Could you check a few things on this model? Use its own coordinates, in mm. Face numbers are marked on the shaded views. A direction names the side the tool comes from. Round coordinates to 2 decimals unless told otherwise and drop trailing zeros. Write each loop counter-clockwise with the first axis right and the second up, starting at its lowest first coordinate (ties: lowest second). Pieces come first, ordered by that corner, then holes. Notation, with made-up numbers: (9, -33.5) -> (31, -33.5) arc R35 cw to (31, 4.5) -> close; hole circle Ø10 at (12.25, 33). An arc over 180 degrees is marked (long way). Answer in a Markdown table with one row per item.
from build123d import *

# Parameters (mm, degrees)
SKETCH1_R           = 3
BOSS_EXTRUDE1_DEPTH = 1
BOSS_EXTRUDE2_DEPTH = 4
SKETCH3_R           = 1.5
BOSS_EXTRUDE3_DEPTH = 8
CHAMFER1_SIZE       = 0.5
SKETCH4_R           = 1.5
CUT_EXTRUDE1_DEPTH  = 3


with BuildPart() as part:
    # Sketch1 → Boss-Extrude1 (new body)
    with BuildSketch(Plane(origin=(0, 0, 0), x_dir=(1, 0, 0), z_dir=(0, 1, 0))):
        with Locations(Location((0, 0, 0), (0, 0, 270))):
            Circle(SKETCH1_R)
    extrude(amount=BOSS_EXTRUDE1_DEPTH)

    # Sketch2 → Boss-Extrude2 (add)
    with BuildSketch(Plane(origin=(0, 1, 0), x_dir=(1, 0, 0), z_dir=(0, 1, 0))):
        Polygon((3.464101615, 0), (1.732050808, 3), (-1.732050808, 3), (-3.464101615, 0), (-1.732050808, -3), (1.732050808, -3), align=None)
    extrude(amount=BOSS_EXTRUDE2_DEPTH)

    # Sketch3 → Boss-Extrude3 (add)
    with BuildSketch(Plane(origin=(0, 5, 0), x_dir=(1, 0, 0), z_dir=(0, 1, 0))):
        with Locations(Location((0, 0, 0), (0, 0, 270))):
            Circle(SKETCH3_R)
    extrude(amount=BOSS_EXTRUDE3_DEPTH)

    # Chamfer1
    chamfer1_edges = [part.edges().sort_by_distance(p)[0] for p in [
        (0, 13, -1.5),
    ]]
    chamfer(chamfer1_edges, length=CHAMFER1_SIZE)

    # Sketch4 → Cut-Extrude1 (cut)
    with BuildSketch(Plane.XZ):
        with Locations(Location((0, 0, 0), (0, 0, 90))):
            Circle(SKETCH4_R)
    extrude(amount=-CUT_EXTRUDE1_DEPTH, mode=Mode.SUBTRACT)


solid = part.part
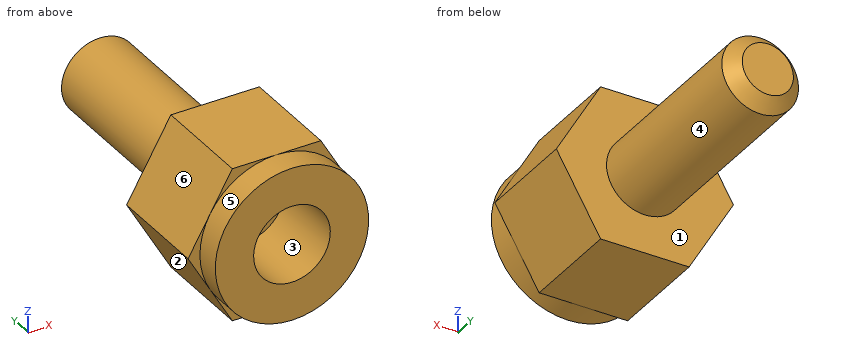
1) Imagine slicing it at D-D, the plane y = 8.5. Please give me the cut outline in (x, z), plus the area to 3 significant figures.
Findings:
| item | result |
|---|---|
| outline | circle Ø3 at (0, 0) |
| area | 7.07 mm^2 |
2) For pin 1 (1.5 mm diameter, centred on x = -1.5, z = -2.5, fed in from +Y), with a flat end and sliding along its axis, tell me the tip position at first contact or that it passes through.
Findings:
| item | result |
|---|---|
| pin 1 | stops at y = 5 |
3) Thinking about a two-plate mould opening in Z: for the marked faces 1, 2 and 3, which applies, +Z half, -Z half, draft (parallel to the pull), parting line (faces both ways), or undercut?
Findings:
| item | result |
|---|---|
| face 1 | draft |
| face 2 | -Z half |
| face 3 | undercut |
4) For the marked faces 4, 5 and 6, which set-ups out of +Z, -Z, +X, -X, +Y, -Y let a thin tool reach every point of the face, with its end or its side?
Findings:
| item | result |
|---|---|
| face 4 | +Y |
| face 5 | -Y |
| face 6 | +Z, -X, +Y, -Y |
5) Please list where these lines run through material, in increasing order: line 1 (X direction, y = 0.75, z = 0); line 2 (Y direction, x = 0, z = 0.5); line 3 (Y direction, x = -1, z = 1.75).
Findings:
| item | result |
|---|---|
| line 1 | x = -3 to -1.5, 1.5 to 3 |
| line 2 | y = 3 to 13 |
| line 3 | y = 0 to 5 |
6) Imagine slicing it at A-A, the plane y = 4. Please give me the cut outline in (x, z), plus the area to 3 significant figures.
Findings:
| item | result |
|---|---|
| outline | (-3.46, 0) -> (-1.73, -3) -> (1.73, -3) -> (3.46, 0) -> (1.73, 3) -> (-1.73, 3) -> close |
| area | 31.2 mm^2 |
7) Imagine slicing it at B-B, the plane z = -2.5. Please give me the cut outline in (x, y), plus the area to 3 significant figures.
Findings:
| item | result |
|---|---|
| outline | (-2.02, 1) -> (-1.66, 1) -> (-1.66, 0) -> (1.66, 0) -> (1.66, 1) -> (2.02, 1) -> (2.02, 5) -> (-2.02, 5) -> close |
| area | 19.5 mm^2 |
8) Imagine slicing it at C-C, the plane z = 2. Please give me the cut outline in (x, y), plus the area to 3 significant figures.
Findings:
| item | result |
|---|---|
| outline | (-2.31, 1) -> (-2.24, 1) -> (-2.24, 0) -> (2.24, 0) -> (2.24, 1) -> (2.31, 1) -> (2.31, 5) -> (-2.31, 5) -> close |
| area | 22.9 mm^2 |
